from build123d import *

# Parameters (mm, degrees)
SKETCH1_W                      = 80
SKETCH1_H                      = 400
BOSS_EXTRUDE1_DEPTH            = 18
FILLET1_R                      = 50
CBORE_FOR_M5_SHCS1_D           = 5.5
CBORE_FOR_M5_SHCS1_DEPTH       = 28.347633298
CBORE_FOR_M5_SHCS1_CBORE_D     = 10
CBORE_FOR_M5_SHCS1_CBORE_DEPTH = 5
CBORE_FOR_M5_SHCS1_TIP         = 1.652366702
CHAMFER1_SIZE                  = 1
SKETCH5_R                      = 3.25
CUT_EXTRUDE1_DEPTH             = 284.418418597
CHAMFER2_SIZE                  = 1


with BuildPart() as part:
    # Sketch1 → Boss-Extrude1 (new body)
    with BuildSketch(Plane.XY):
        with Locations((41, 71)):
            Rectangle(SKETCH1_W, SKETCH1_H)
    extrude(amount=BOSS_EXTRUDE1_DEPTH)

    # Fillet1
    fillet1_edges = [part.edges().sort_by_distance(p)[0] for p in [
        (81, 271, 9),
        (81, -129, 9),
    ]]
    fillet(fillet1_edges, radius=FILLET1_R)

    # CBORE for M5 SHCS1
    with Locations(Plane.XY.offset(18)):
        with Locations((9.25, 190), (9.25, 130), (9.25, 70), (9.25, 10), (9.25, -50), (9.25, -110), (9.25, 250)):
            CounterBoreHole(CBORE_FOR_M5_SHCS1_D / 2, CBORE_FOR_M5_SHCS1_CBORE_D / 2, CBORE_FOR_M5_SHCS1_CBORE_DEPTH, depth=CBORE_FOR_M5_SHCS1_DEPTH)
            with Locations((0, 0, -(CBORE_FOR_M5_SHCS1_DEPTH + CBORE_FOR_M5_SHCS1_TIP / 2))):  # 118° drill point
                Cone(0, CBORE_FOR_M5_SHCS1_D / 2, CBORE_FOR_M5_SHCS1_TIP, mode=Mode.SUBTRACT)

    # Chamfer1
    chamfer1_edges = [part.edges().sort_by_distance(p)[0] for p in [
        (16, 271, 18),
        (81, 71, 18),
        (66.355339059, -114.355339059, 18),
        (66.355339059, 256.355339059, 18),
        (4.25, 250, 18),
        (4.25, -110, 18),
        (4.25, -50, 18),
        (1, 71, 18),
        (4.25, 10, 18),
        (4.25, 70, 18),
        (4.25, 130, 18),
        (4.25, 190, 18),
        (16, -129, 18),
    ]]
    chamfer(chamfer1_edges, length=CHAMFER1_SIZE)

    # Sketch5 → Cut-Extrude1 (cut, through all)
    with BuildSketch(Plane.XY.offset(18)):
        with Locations((29.25, 40)):
            Circle(SKETCH5_R)
    extrude(amount=-CUT_EXTRUDE1_DEPTH, mode=Mode.SUBTRACT)

    # Chamfer2
    chamfer2_edges = [part.edges().sort_by_distance(p)[0] for p in [
        (26, 40, 0),
        (26, 40, 18),
    ]]
    chamfer(chamfer2_edges, length=CHAMFER2_SIZE)


solid = part.part
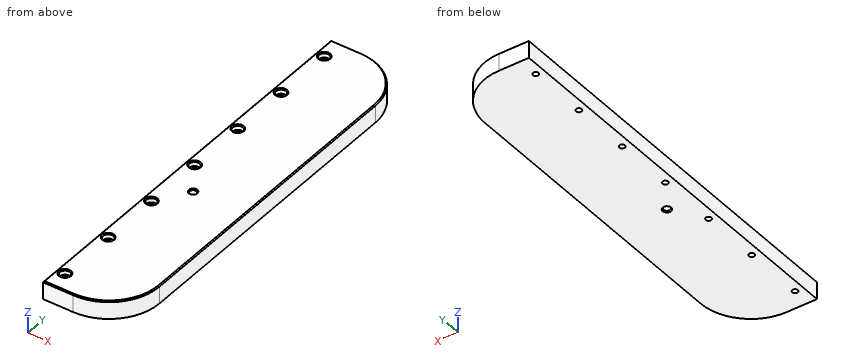
Here's how the part is built. I have some questions about the finished solid (model axes, mm). Coordinates: 2 decimals unless noted, no trailing zeros.
Item 1: I need wall thicknesses on line 1 (X direction, y = 190, z = 9.25); line 2 (Y direction, x = 29.5, z = 15.75); line 3 (Y direction, x = 41, z = 14.5). Which ranges of each line are inside material? Lowest first, please.
Result sheet:
line 1: x = 1 to 6.5, 12 to 81
line 2: y = -129 to 36.76, 43.24 to 271
line 3: y = -127.99 to 269.99
Item 2: For P1, Ø1.5, axis at x = 43.5, z = 4, coming from the -Y side; P2, Ø9, axis at x = 9.25, y = 70, coming from the +Z side; P3, Ø1.5, axis at x = 38, z = 12.5, coming from the -Y side, each with a flat end and sliding along its axis, tell me the tip position at first contact or that it passes through.
Result sheet:
P1: stops at y = -127.6
P2: stops at z = 13
P3: stops at y = -128.61
Item 3: If we section it at A-A on z = 10: State how many separate pieces and enclosed holes the cut face has, plus the area to 3 significant figures.
Result sheet:
separate pieces: 1
enclosed holes: 8
area: 30,700 mm2
